Design review of the part built by this model. Coordinates are the model's own, in mm. A direction names the side the tool comes from. Coordinates: 2 decimals unless noted, no trailing zeros. Loops run counter-clockwise (first coordinate to the right, second up) from the corner with the lowest first, then second, coordinate; pieces in that order, holes last. Notation, with made-up numbers: (-35, -9.75) -> (-8, -9.75) arc R29 cw to (-8, 14.25) -> close; hole circle Ø4 at (-27, 56). An arc over 180 degrees is marked (long way). Use a Markdown table: item, result. Add a question column.
Q1. Take a section at A-A on z = -133. Write out the cut boundary in (x, y).
Q2. Clearance check with flat-ended pins moving along their axes: pin 1 Ø1.5 at (x, y) = (31.5, -1) entering from +Z; pin 2 Ø0.9 at (y, z) = (-1.5, -150) entering from -X; pin 3 Ø1.5 at (y, z) = (-1, -150) entering from +X. State where each tip first meets the part, or that it passes through.
Q3. Draft analysis for pull direction X (two halves, no side actions). For faces 1 (the face through (24, -1, -100)), 2 (the face through (-1, -3, -73)), state which applies: pulls with the +X half, pulls with the -X half, needs draft (parallel to the pull), parting line crosses it, or undercut.
Q4. Take a section at C-C on x = 7. Write out the cut boundary in (y, z), plus the area to 3 significant figures.
Q5. Take a section at B-B on y = -1.95. Count the separate pieces of the cut face and the enclosed holes in it, plus the area to 3 significant figures.
Q6. Take a section at D-D on x = -52. Write out the cut boundary in (y, z).
Q7. For faces 3 (the face through (-25, -1, -101)), 4 (the face through (-1, 0, -73)), list the 3-axis set-ups (+Z, -Z, +X, -X, +Y, -Y) from which the entire face can be reached by the end or side of a thin tool; tool diameter is ignored.
Q8. For probe 1 along X at (y, z) = (-0.65, -135); probe 2 along Z at (x, y) = (29, -2.9); probe 3 along Z at (x, y) = (-17, -1.9), list the stretches that pass through material, from the lowest coordinate up.
from build123d import *

# Parameters (mm, degrees)
F1_W     = 8
F1_H     = 3.1
F2_DEPTH = 3


with BuildPart() as f2:
    # F1 (on Front) → F2 (new body)
    with BuildSketch(Plane.XZ):
        with BuildLine():
            Line((82, 0), (82, 3))
            Line((82, 3), (75, 3))
            Line((75, 3), (75, 0))
            Line((75, 0), (65, 0))
            Line((65, 0), (65, 3))
            Line((65, 3), (55, 3))
            Line((55, 3), (55, 0))
            Line((55, 0), (45, 0))
            Line((45, 0), (45, 3))
            Line((45, 3), (35, 3))
            Line((35, 3), (35, 0))
            Line((35, 0), (25, 0))
            Line((25, 0), (25, 3))
            Line((25, 3), (15, 3))
            Line((15, 3), (15, 0))
            Line((15, 0), (5, 0))
            Line((5, 0), (5, 3))
            Line((5, 3), (-5, 3))
            Line((-5, 3), (-5, 0))
            Line((-5, 0), (-15, 0))
            Line((-15, 0), (-15, 3))
            Line((-15, 3), (-25, 3))
            Line((-25, 3), (-25, 0))
            Line((-25, 0), (-35, 0))
            Line((-35, 0), (-35, 3))
            Line((-35, 3), (-45, 3))
            Line((-45, 3), (-45, 0))
            Line((-45, 0), (-55, 0))
            Line((-55, 0), (-55, 3))
            Line((-55, 3), (-65, 3))
            Line((-65, 3), (-65, 0))
            Line((-65, 0), (-75, 0))
            Line((-75, 0), (-75, 3))
            Line((-75, 3), (-82, 3))
            Line((-82, 3), (-82, 0))
            Line((-82, 0), (-85, 0))
            Line((-85, 0), (-85, -10))
            Line((-85, -10), (-82, -10))
            Line((-82, -10), (-82, -20))
            Line((-82, -20), (-85, -20))
            Line((-85, -20), (-85, -30))
            Line((-85, -30), (-82, -30))
            Line((-82, -30), (-82, -40))
            Line((-82, -40), (-85, -40))
            Line((-85, -40), (-85, -50))
            Line((-85, -50), (-82, -50))
            Line((-82, -50), (-82, -60))
            Line((-82, -60), (-85, -60))
            Line((-85, -60), (-85, -70))
            Line((-85, -70), (-82, -70))
            Line((-82, -70), (-82, -80))
            Line((-82, -80), (-85, -80))
            Line((-85, -80), (-85, -90))
            Line((-85, -90), (-82, -90))
            Line((-82, -90), (-82, -100))
            Line((-82, -100), (-85, -100))
            Line((-85, -100), (-85, -110))
            Line((-85, -110), (-82, -110))
            Line((-82, -110), (-82, -120))
            Line((-82, -120), (-85, -120))
            Line((-85, -120), (-85, -130))
            Line((-85, -130), (-82, -130))
            Line((-82, -130), (-82, -140))
            Line((-82, -140), (-85, -140))
            Line((-85, -140), (-85, -149))
            Line((-85, -149), (-75, -149))
            Line((-75, -149), (-75, -152))
            Line((-75, -152), (-65, -152))
            Line((-65, -152), (-65, -149))
            Line((-65, -149), (-55, -149))
            Line((-55, -149), (-55, -152))
            Line((-55, -152), (-45, -152))
            Line((-45, -152), (-45, -149))
            Line((-45, -149), (-26, -149))
            Line((-26, -149), (-26, -113))
            Line((-26, -113), (-34, -113))
            Line((-34, -113), (-34, -109.9))
            Line((-34, -109.9), (-26, -109.9))
            Line((-26, -109.9), (-26, -104))
            ThreePointArc((-26, -104), (-24.535534, -100.464466), (-21, -99))
            Line((-21, -99), (21, -99))
            ThreePointArc((21, -99), (24.535534, -100.464466), (26, -104))
            Line((26, -104), (26, -109.9))
            Line((26, -109.9), (34, -109.9))
            Line((34, -109.9), (34, -113))
            Line((34, -113), (26, -113))
            Line((26, -113), (26, -149))
            Line((26, -149), (45, -149))
            Line((45, -149), (45, -152))
            Line((45, -152), (55, -152))
            Line((55, -152), (55, -149))
            Line((55, -149), (65, -149))
            Line((65, -149), (65, -152))
            Line((65, -152), (75, -152))
            Line((75, -152), (75, -149))
            Line((75, -149), (85, -149))
            Line((85, -149), (85, -140))
            Line((85, -140), (82, -140))
            Line((82, -140), (82, -130))
            Line((82, -130), (85, -130))
            Line((85, -130), (85, -120))
            Line((85, -120), (82, -120))
            Line((82, -120), (82, -110))
            Line((82, -110), (85, -110))
            Line((85, -110), (85, -100))
            Line((85, -100), (82, -100))
            Line((82, -100), (82, -90))
            Line((82, -90), (85, -90))
            Line((85, -90), (85, -80))
            Line((85, -80), (82, -80))
            Line((82, -80), (82, -70))
            Line((82, -70), (85, -70))
            Line((85, -70), (85, -60))
            Line((85, -60), (82, -60))
            Line((82, -60), (82, -50))
            Line((82, -50), (85, -50))
            Line((85, -50), (85, -40))
            Line((85, -40), (82, -40))
            Line((82, -40), (82, -30))
            Line((82, -30), (85, -30))
            Line((85, -30), (85, -20))
            Line((85, -20), (82, -20))
            Line((82, -20), (82, -10))
            Line((82, -10), (85, -10))
            Line((85, -10), (85, 0))
            Line((85, 0), (82, 0))
        make_face()
        with Locations((-46, -111.45)):
            Rectangle(F1_W, F1_H, mode=Mode.SUBTRACT)
        with Locations((46, -111.45)):
            Rectangle(F1_W, F1_H, mode=Mode.SUBTRACT)
    extrude(amount=F2_DEPTH)


solid = f2.part
Answer list:
| question | item | result |
|---|---|---|
| 1 | outline | (-82, -3) -> (-26, -3) -> (-26, 0) -> (-82, 0) -> close; (26, -3) -> (82, -3) -> (82, 0) -> (26, 0) -> close |
| 2 | pin 1 | z = 0 |
| 2 | pin 2 | x = -75 |
| 2 | pin 3 | x = 75 |
| 3 | face 1 | undercut |
| 3 | face 2 | needs draft |
| 4 | outline | (-3, -99) -> (0, -99) -> (0, 0) -> (-3, 0) -> close |
| 4 | area | 297 mm² |
| 5 | separate pieces | 1 |
| 5 | enclosed holes | 2 |
| 5 | area | 22,600 mm² |
| 6 | outline | (-3, -152) -> (0, -152) -> (0, 0) -> (-3, 0) -> close |
| 7 | face 3 | -Z, +Y, -Y |
| 7 | face 4 | +Z, -Z, +X, -X, +Y |
| 8 | probe 1 | -82 to -26, 26 to 82 |
| 8 | probe 2 | -149 to -113, -109.9 to 0 |
| 8 | probe 3 | -99 to 3 |
